from build123d import *

# Parameters (mm, degrees)
F1_DEPTH = 8
F2_R     = 5
F3_DEPTH = 8.001
F4_R     = 6
F5_DEPTH = 5
F7_D     = 6.6
F8_R     = 3.125
F9_DEPTH = 8.001


with BuildPart() as f1:
    # F0 (on Top) → F1 (new body)
    with BuildSketch(Plane.XY):
        with BuildLine():
            ThreePointArc((-28.3169756085, -7.8291564448), (-27.7311891708, -9.2433700072), (-26.3169756085, -9.8291564448))
            Line((-26.3169756085, -9.8291564448), (14.6830243915, -9.8291564448))
            ThreePointArc((14.6830243915, -9.8291564448), (16.0972379539, -9.2433700072), (16.6830243915, -7.8291564448))
            Line((16.6830243915, -7.8291564448), (16.6830243915, 14.1708435552))
            ThreePointArc((16.6830243915, 14.1708435552), (16.0972379539, 15.5850571176), (14.6830243915, 16.1708435552))
            Line((14.6830243915, 16.1708435552), (-17.4885484837, 16.1708435552))
            ThreePointArc((-17.4885484837, 16.1708435552), (-18.2539153485, 16.0186026202), (-18.9027620461, 15.5850571176))
            Line((-18.9027620461, 15.5850571176), (-27.7311891708, 6.7566299928))
            ThreePointArc((-27.7311891708, 6.7566299928), (-28.1647346735, 6.1077832952), (-28.3169756085, 5.3424164305))
            Line((-28.3169756085, 5.3424164305), (-28.3169756085, -7.8291564448))
        make_face()
    extrude(amount=F1_DEPTH)

    # F2 (on face) → F3 (cut, through all)
    with BuildSketch(Plane.XY.offset(8)):
        with Locations((1.6830243915, -1.8291564448)):
            Circle(F2_R)
    extrude(amount=-F3_DEPTH, mode=Mode.SUBTRACT)

    # F4 (on face) → F5 (cut)
    with BuildSketch(Plane.XY.offset(8)):
        with Locations((1.6830243915, -1.8291564448)):
            Circle(F4_R)
    extrude(amount=-F5_DEPTH, mode=Mode.SUBTRACT)

    # F7 (through all)
    with Locations(Plane.XY.offset(8)):
        with Locations((-9.3169756085, 11.1708435552), (8.6830243915, 11.1708435552)):
            Hole(F7_D / 2)

    # F8 (on face) → F9 (cut, through all)
    with BuildSketch(Plane.XY.offset(8)):
        with Locations((-21.5339642018, -3.0962659512)):
            Circle(F8_R)
    extrude(amount=-F9_DEPTH, mode=Mode.SUBTRACT)


solid = f1.part
Input: part model. Units: mm. Frame: model coordinates. A direction names the side the tool comes from. Coordinates: 2 decimals unless noted, no trailing zeros. Order: outer loops, then holes, each group sorted by start corner. A loop starts at its lowest first (then second) coordinate and runs counter-clockwise, first axis right, second up. Notation, with made-up numbers: M 4,58.5 L 59,58.5 A19 ccw 59,77.5 Z; hole C 2,-8.5 d11. An arc over 180 degrees is marked long. Write item = value, one per line. Start each with the question number.
(1) Pull-direction query (Y, two-part tool) for faces 3 (the flat face through (-6, 3, 8)), 4 (the cylindrical face through (6.452, -0.327, 1.521)), 5 (the cylindrical face through (-18.244, 16.023, 3.944)); classes: released by +Y, released by -Y, zero draft, split by the parting line, or undercut.
(2) Section D-D on y = -4.75. Output: boundary loops of the cut face in (x, z).
(3) Section C-C on z = 5. Output: boundary loops of the cut face in (x, y) (3 decimals), and give its area (3 significant figures).
(4) Line query: line 1 along X through (y, z) = (1.5, 4.25); line 2 along Y through (x, z) = (6, 7.5); line 3 along X through (y, z) = (-3.5, 5.5). Output: solid intervals per line, ascending. Write a range as [from, to].
(5) Section B-B on x = -7. Output: boundary loops of the cut face in (y, z), and give its area (3 significant figures).
(6) Reachability of faces 1 (the cylindrical face through (-6.7, 9.16, 3.94)), 2 (the cylindrical face through (7.406, -0.027, 5.535)) from +Z, -Z, +X, -X, +Y, -Y: full face, straight path, thin tool, end or side. Return the list, or none.
(7) Section A-A on y = 0.75. Output: boundary loops of the cut face in (x, z).
(8) First-contact query: P1, Ø2, axis at x = -22, z = 1, coming from the +Y side. Flat tip, straight axial feed; report the tip coordinate or a pass-through.
Result set:
q1.face_3 = zero draft
q1.face_4 = undercut
q1.face_5 = released by +Y
q2.outline = M -28.32,0 L -24.19,0 L -24.19,8 L -28.32,8 Z; M -18.88,0 L -2.38,0 L -2.38,3 L -3.56,3 L -3.56,8 L -18.88,8 Z; M 5.74,0 L 16.68,0 L 16.68,8 L 6.92,8 L 6.92,3 L 5.74,3 Z
q3.outline = M -28.317,-7.829 A2 ccw -26.317,-9.829 L 14.683,-9.829 A2 ccw 16.683,-7.829 L 16.683,14.171 A2 ccw 14.683,16.171 L -17.489,16.171 A2 ccw -18.903,15.585 L -27.731,6.757 A2 ccw -28.317,5.342 Z; hole C -21.534,-3.096 d6.25; hole C -9.317,11.171 d6.6; hole C 1.683,-1.829 d12; hole C 8.683,11.171 d6.6
q3.area = 905 mm²
q4.line_1 = [-28.32, -3.31], [6.67, 16.68]
q4.line_2 = [-9.83, -6], [2.34, 9.25], [13.09, 16.17]
q4.line_3 = [-28.32, -24.63], [-18.44, -4.08], [7.45, 16.68]
q5.outline = M -9.83,0 L 8.82,0 L 8.82,8 L -9.83,8 Z; M 13.52,0 L 16.17,0 L 16.17,8 L 13.52,8 Z
q5.area = 170 mm²
q6.face_1 = +Z, -Z
q6.face_2 = +Z
q7.outline = M -28.32,0 L -2.6,0 L -2.6,3 L -3.73,3 L -3.73,8 L -28.32,8 Z; M 5.97,0 L 16.68,0 L 16.68,8 L 7.1,8 L 7.1,3 L 5.97,3 Z
q8.P1 = 13.49
